The model under review builds one solid part; all positions refer to its coordinate system, in mm. A direction names the side the tool comes from. Round coordinates to 2 decimals unless told otherwise and drop trailing zeros. Write each loop counter-clockwise with the first axis right and the second up, starting at its lowest first coordinate (ties: lowest second). Pieces come first, ordered by that corner, then holes. Notation, with made-up numbers: M 14,77.5 L 72,77.5 A8 cw 72,88.5 Z; hole C 18,7.5 d4. An arc over 180 degrees is marked long. One line per item, written item: value. Start each with the question number.
1) Take a section at B-B, the plane x = 0. Write out the cut boundary in (y, z), and give its area (3 significant figures).
2) Take a section at C-C, the plane y = 21.5. Write out the cut boundary in (x, z).
3) Take a section at A-A, the plane z = 0. Write out the cut boundary in (x, y).
4) Tool access review of faces 1 (the face through (0, 0, 0)), 2 (the face through (3.1, 52.2, 0.7)): name each direction out of +Z, -Z, +X, -X, +Y, -Y from which nothing blocks a thin tool from reaching the whole face with its end or side.
5) Wall thickness on probe 1 along Y at (x, z) = (-3.5, -22); probe 2 along Y at (x, z) = (-13, -20.5); probe 3 along X at (y, z) = (5, -2.5): over which ranges is each line inside the solid? List them lowest first.
6) For P1, Ø24, axis at x = -9.5, z = -11.5, coming from the +Y side; P2, Ø1, axis at x = 4.5, y = 12.5, coming from the +Z side; P3, Ø4, axis at y = 11, z = -10, coming from the -X side; P4, Ø10, axis at x = -3, z = -18.5, coming from the +Y side, all flat-tipped, find the tip position at first contact; note any pin that passes through.
from build123d import *

# Parameters (mm, degrees)
FILLET1_R     = 15.25
CHAMFER1_SIZE = 1


with BuildPart() as part:
    # Sketch1 → Revolve1 (revolve)
    with BuildSketch(Plane.XY, mode=Mode.PRIVATE) as revolve1_sk:
        Polygon((0, 0), (-26.67, 0), (-26.67, 1.27), (-24.131486656, 3.808513344), (-3.18, 3.808513344), (-3.18, 85.408513344), (0, 85.408513344), align=None)
    revolve(revolve1_sk.sketch.rotate(Axis((0, 0, 0), (0, 1, 0)), 270), axis=Axis((0, 0, 0), (0, 1, 0)))

    # Fillet1
    fillet1_edges = [part.edges().sort_by_distance(p)[0] for p in [
        (0, 3.808513344, 3.18),
    ]]
    fillet(fillet1_edges, radius=FILLET1_R)

    # Chamfer1
    chamfer1_edges = [part.edges().sort_by_distance(p)[0] for p in [
        (0, 85.408513344, 3.18),
    ]]
    chamfer(chamfer1_edges, length=CHAMFER1_SIZE)


solid = part.part
Checked values:
1. outline: M 0,-26.67 L 1.27,-26.67 L 3.81,-24.13 L 3.81,-18.43 A15.25 cw 19.06,-3.18 L 84.41,-3.18 L 85.41,-2.18 L 85.41,2.18 L 84.41,3.18 L 19.06,3.18 A15.25 cw 3.81,18.43 L 3.81,24.13 L 1.27,26.67 L 0,26.67 Z
1. area: 814 mm2
2. outline: C 0,0 d6.36
3. outline: M -26.67,0 L 26.67,0 L 26.67,1.27 L 24.13,3.81 L 18.43,3.81 A15.25 cw 3.18,19.06 L 3.18,84.41 L 2.18,85.41 L -2.18,85.41 L -3.18,84.41 L -3.18,19.06 A15.25 cw -18.43,3.81 L -24.13,3.81 L -26.67,1.27 Z
4. face 1: +Z, -Z, +X, -X, -Y
4. face 2: +Y
5. probe 1: y = 0 to 3.81
5. probe 2: y = 0 to 3.67
5. probe 3: x = -12.27 to 12.27
6. P1: stops at y = 84.67
6. P2: stops at z = 2.52
6. P3: passes through
6. P4: stops at y = 4.55
